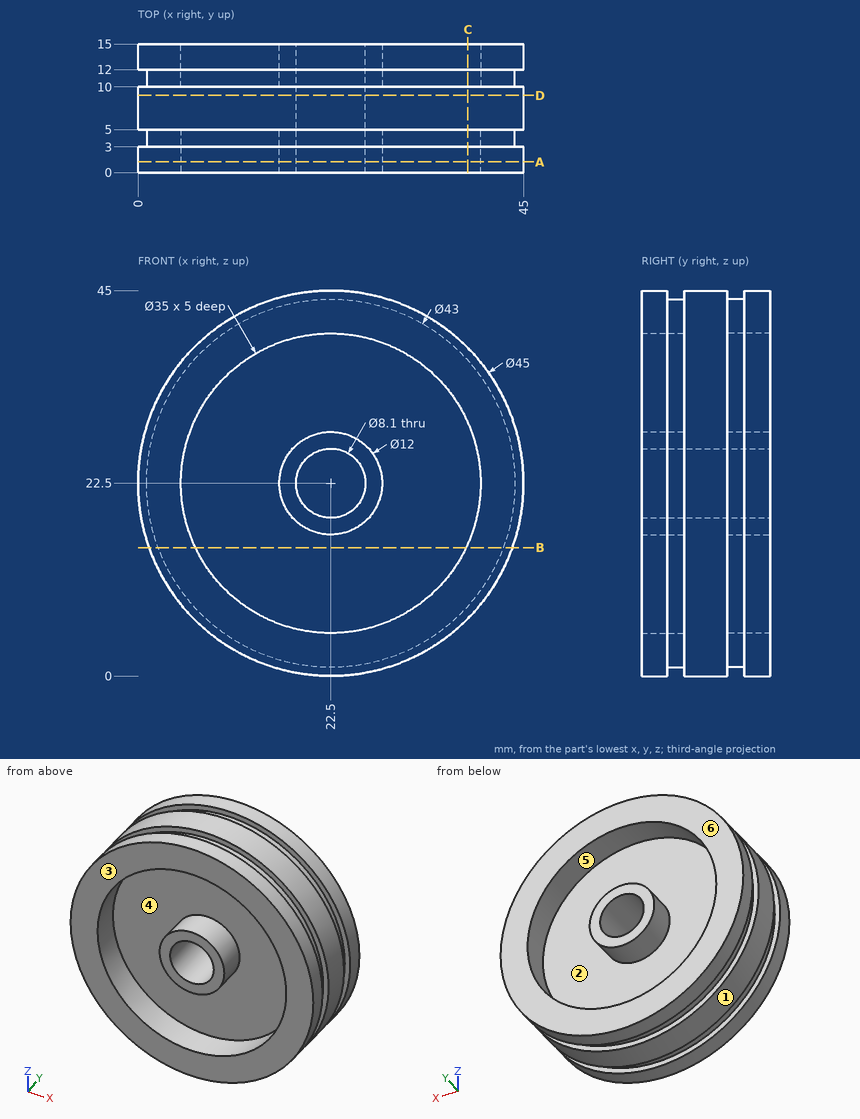
Study the drawing (mm; zero at the part's minimum x, y, z) and answer. A direction names the side the tool comes from. Coordinates: 2 decimals unless noted, no trailing zeros. Write each loop counter-clockwise with the first axis right and the second up, starting at its lowest first coordinate (ties: lowest second). Pieces come first, ordered by that corner, then holes. Notation, with made-up numbers: M 82,88 L 134,88 A11 cw 134,103 Z; hole C 12.5,82.5 d11. An arc over 180 degrees is marked long. Use one line per item in the form item = value.
Item 1: Find section A-A, the plane y = 1.25. Give the vertices of the cut face in (x, z).
Model answer:
outline = C 22.5,22.5 d45; C 22.5,22.5 d12; hole C 22.5,22.5 d35; hole C 22.5,22.5 d8.1
Item 2: For the marked faces 4, 5 and 6, determine the directions among +Z, -Z, +X, -X, +Y, -Y from which every point of the face is accessible in a straight line to the end or side of a thin tool.
Model answer:
face_4 = -Y
face_5 = +Y
face_6 = +Z, -Z, +X, -X, +Y
Item 3: Find section C-C, the plane x = 38.5. Give the vertices of the cut face in (y, z).
Model answer:
outline = M 0,6.68 L 3,6.68 L 3,8.14 L 5,8.14 L 5,6.68 L 10,6.68 L 10,8.14 L 12,8.14 L 12,6.68 L 15,6.68 L 15,15.41 L 10,15.41 L 10,29.59 L 15,29.59 L 15,38.32 L 12,38.32 L 12,36.86 L 10,36.86 L 10,38.32 L 5,38.32 L 5,36.86 L 3,36.86 L 3,38.32 L 0,38.32 L 0,29.59 L 5,29.59 L 5,15.41 L 0,15.41 Z
Item 4: Find section D-D, the plane y = 9. Give the vertices of the cut face in (x, z).
Model answer:
outline = C 22.5,22.5 d45; hole C 22.5,22.5 d8.1
Item 5: The mould has two halves that part along X. Classify the marked faces 1, 2 and 3: released by +X, released by -X, zero draft, split by the parting line, or undercut.
Model answer:
face_1 = split by the parting line
face_2 = undercut
face_3 = zero draft
Item 6: Find the intervals of material crossed by probe 1 along Z at (x, y) = (22.5, 11.8); probe 2 along Z at (x, y) = (22.5, 2.05); probe 3 along Y at (x, z) = (39, 37.5), in increasing order.
Model answer:
probe_1 = 1 to 5, 16.5 to 18.45, 26.55 to 28.5, 40 to 44
probe_2 = 0 to 5, 16.5 to 18.45, 26.55 to 28.5, 40 to 45
probe_3 = 0 to 3, 5 to 10, 12 to 15
Item 7: Find section B-B, the plane z = 15. Give the vertices of the cut face in (x, y), plus the area to 3 significant figures.
Model answer:
outline = M 1.29,0 L 6.69,0 L 6.69,5 L 38.31,5 L 38.31,0 L 43.71,0 L 43.71,3 L 42.65,3 L 42.65,5 L 43.71,5 L 43.71,10 L 42.65,10 L 42.65,12 L 43.71,12 L 43.71,15 L 38.31,15 L 38.31,10 L 6.69,10 L 6.69,15 L 1.29,15 L 1.29,12 L 2.35,12 L 2.35,10 L 1.29,10 L 1.29,5 L 2.35,5 L 2.35,3 L 1.29,3 Z
area = 312 mm2
Item 8: Given P1, Ø4, axis at x = 8, y = 10, coming from the +Z side; P2, Ø2, axis at y = 12, z = 11, coming from the +X side; P3, Ø5, axis at y = 4, z = 16.5, coming from the -X side, each flat-ended and moving along its own axis, determine where each tip first touches the part or whether it passes through.
Model answer:
P1 = 41.21
P2 = 42.4
P3 = 0.31
